Source: three-view drawing plus pictorial views. Frame: mm from the lowest corner of the part. A direction names the side the tool comes from. Round coordinates to 2 decimals unless told otherwise and drop trailing zeros. Order: outer loops, then holes, each group sorted by start corner. A loop starts at its lowest first (then second) coordinate and runs counter-clockwise, first axis right, second up. Notation, with made-up numbers: (21, 31) - (30, 31) arc R7 ccw to (30, 35) - close; hole circle Ø2 at (1, 79.5). An arc over 180 degrees is marked (long way). Use one line per item in the form item = value. Start each with the question number.
Q1. Set-up query: the marked faces 1 and 2. Return all of +Z, -Z, +X, -X, +Y, -Y with unobstructed straight access to the full face (end or side cutting, diameter ignored); none if empty.
Q2. Cut plane C-C, the plane x = 4.25. Return the cut outline in (y, z).
Q3. Cut plane A-A, the plane y = 14.3. Return the cut outline in (x, z), and give its area (3 significant figures).
Q4. Ray query, line 1 (Y direction, x = 4.5, z = 14.3); line 2 (X direction, y = 16.5, z = 23.25). Return the intervals inside material, ascending. Write a range as [from, to].
Q5. Pin query (flat end, axial travel): pin 1 Ø1.5 at (y, z) = (21, 7.5) entering from -X; pin 2 Ø6 at (y, z) = (5, 20.5) entering from +X; pin 3 Ø1.5 at (x, y) = (4, 10.5) entering from -Z; pin 4 Ø2.5 at (y, z) = (14.3, 14.3) entering from +X (3 decimals). Return the tip coordinate at first contact, or that it passes through.
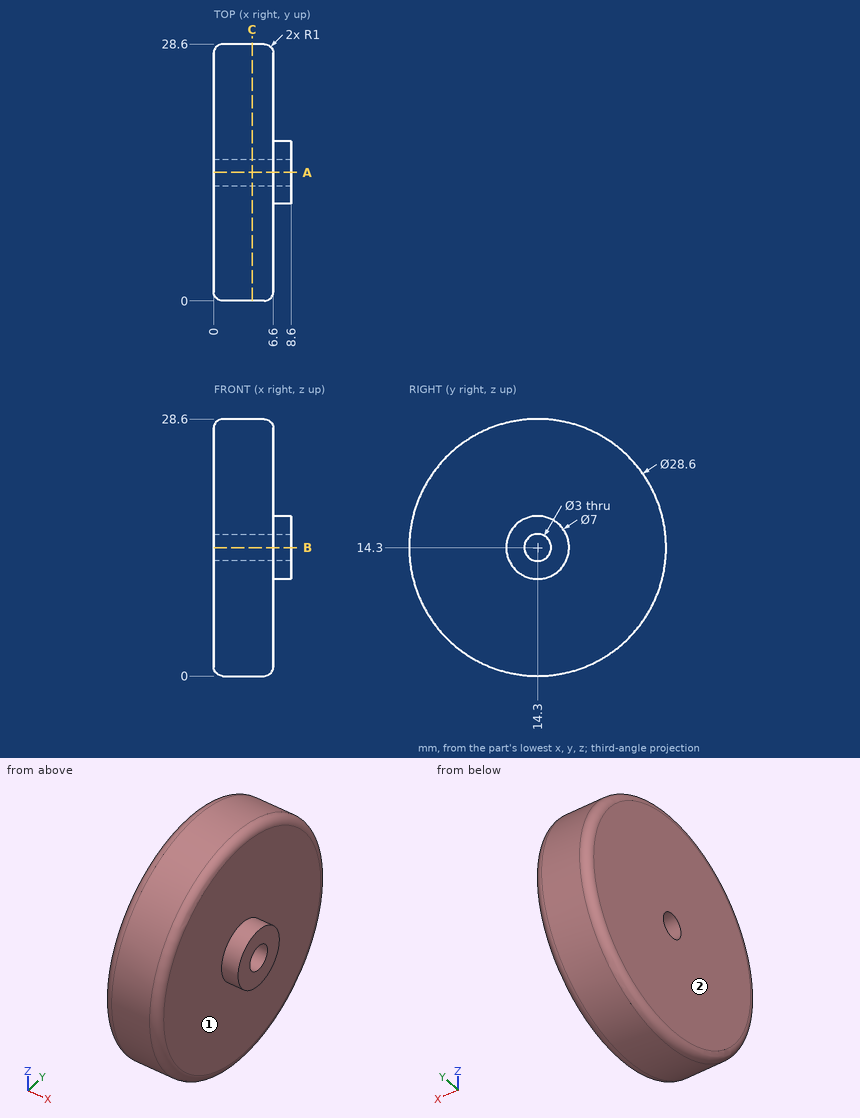
Completed:
q1.face_1 = +X
q1.face_2 = +Z, -Z, -X, +Y, -Y
q2.outline = circle Ø28.6 at (14.3, 14.3); hole circle Ø3 at (14.3, 14.3)
q3.outline = (0, 1) arc R1 ccw to (1, 0) - (5.6, 0) arc R1 ccw to (6.6, 1) - (6.6, 10.8) - (8.6, 10.8) - (8.6, 12.8) - (0, 12.8) - close; (0, 15.8) - (8.6, 15.8) - (8.6, 17.8) - (6.6, 17.8) - (6.6, 27.6) arc R1 ccw to (5.6, 28.6) - (1, 28.6) arc R1 ccw to (0, 27.6) - close
q3.area = 176 mm2
q4.line_1 = [0, 12.8], [15.8, 28.6]
q4.line_2 = [0, 6.6]
q5.pin_1 = 0
q5.pin_2 = 6.6
q5.pin_3 = 0.33
q5.pin_4 = through
